```python
from build123d import *

# Parameters (mm, degrees)
SKETCH1_W           = 24.999989911
SKETCH1_H           = 10.457138345
SKETCH1_W_2         = 49.999979697
SKETCH1_H_2         = 10.999995004
BOSS_EXTRUDE1_DEPTH = 6


with BuildPart() as part:
    # Sketch1 → Boss-Extrude1 (new body)
    with BuildSketch(Plane.XY):
        Polygon((-65.562023318, 106.501824812), (-13.869587203, 106.501824812), (-8.869589203, 111.501822737), (-8.86958929, 177.416081581), (-13.869587182, 182.416079474), (-65.562023318, 182.416079474), (-70.562021318, 177.416081474), (-70.562021318, 111.501822812), align=None)
        with Locations((-39.715805178, 122.080389652)):
            Rectangle(SKETCH1_W, SKETCH1_H, mode=Mode.SUBTRACT)
        with Locations((-39.715804889, 167.108942347)):
            Rectangle(SKETCH1_W_2, SKETCH1_H_2, mode=Mode.SUBTRACT)
        Polygon((-64.027895413, 142.720286351), (-63.562021318, 142.658952863), (-63.096147223, 142.720286351), (-62.662021678, 142.90010704), (-62.289229621, 143.186160446), (-62.003176215, 143.558952503), (-61.823355526, 143.993078048), (-61.762022038, 144.458952143), (-61.823355526, 144.924826238), (-62.003176215, 145.358951783), (-62.289229621, 145.73174384), (-62.662021678, 146.017797246), (-63.096147223, 146.197617935), (-63.562021318, 146.258951423), (-64.027895413, 146.197617935), (-64.462020958, 146.017797246), (-64.834813015, 145.73174384), (-65.120866421, 145.358951783), (-65.30068711, 144.924826238), (-65.362020598, 144.458952143), (-65.30068711, 143.993078048), (-65.120866421, 143.558952503), (-64.834813015, 143.186160446), (-64.462020958, 142.90010704), align=None, mode=Mode.SUBTRACT)
        Polygon((-15.869589241, 146.258951423), (-16.335463335, 146.197617935), (-16.769588881, 146.017797246), (-17.142380938, 145.73174384), (-17.428434344, 145.358951783), (-17.608255032, 144.924826238), (-17.669588521, 144.458952143), (-17.608255032, 143.993078048), (-17.428434344, 143.558952503), (-17.142380938, 143.186160446), (-16.769588881, 142.90010704), (-16.335463335, 142.720286351), (-15.869589241, 142.658952863), (-15.403715146, 142.720286351), (-14.969589601, 142.90010704), (-14.596797544, 143.186160446), (-14.310744137, 143.558952503), (-14.130923449, 143.993078048), (-14.069589961, 144.458952143), (-14.130923449, 144.924826238), (-14.310744137, 145.358951783), (-14.596797544, 145.73174384), (-14.969589601, 146.017797246), (-15.403715146, 146.197617935), align=None, mode=Mode.SUBTRACT)
        Polygon((-37.977139407, 111.967698907), (-38.156960096, 112.401824452), (-38.443013502, 112.774616509), (-38.815805559, 113.060669915), (-39.249931104, 113.240490604), (-39.715805199, 113.301824092), (-40.181679294, 113.240490604), (-40.615804839, 113.060669915), (-40.988596896, 112.774616509), (-41.274650303, 112.401824452), (-41.454470991, 111.967698907), (-41.515804479, 111.501824812), (-41.454470991, 111.035950717), (-41.274650303, 110.601825172), (-40.988596896, 110.229033115), (-40.615804839, 109.942979709), (-40.181679294, 109.76315902), (-39.715805199, 109.701825532), (-39.249931104, 109.76315902), (-38.815805559, 109.942979709), (-38.443013502, 110.229033115), (-38.156960096, 110.601825172), (-37.977139407, 111.035950717), (-37.915805919, 111.501824812), align=None, mode=Mode.SUBTRACT)
        Polygon((-37.977139407, 176.950205359), (-37.915805919, 177.416079454), (-37.977139407, 177.881953549), (-38.156960096, 178.316079094), (-38.443013502, 178.688871151), (-38.815805559, 178.974924557), (-39.249931104, 179.154745246), (-39.715805199, 179.216078734), (-40.181679294, 179.154745246), (-40.615804839, 178.974924557), (-40.988596896, 178.688871151), (-41.274650303, 178.316079094), (-41.454470991, 177.881953549), (-41.515804479, 177.416079454), (-41.454470991, 176.950205359), (-41.274650303, 176.516079814), (-40.988596896, 176.143287757), (-40.615804839, 175.857234351), (-40.181679294, 175.677413662), (-39.715805199, 175.616080174), (-39.249931104, 175.677413662), (-38.815805559, 175.857234351), (-38.443013502, 176.143287757), (-38.156960096, 176.516079814), align=None, mode=Mode.SUBTRACT)
        Polygon((-55.181679294, 134.720286351), (-54.715805199, 134.658952863), (-54.249931104, 134.720286351), (-53.815805559, 134.90010704), (-53.443013502, 135.186160446), (-53.156960096, 135.558952503), (-52.977139407, 135.993078048), (-52.915805919, 136.458952143), (-52.977139407, 136.924826238), (-53.156960096, 137.358951783), (-53.443013502, 137.73174384), (-53.815805559, 138.017797246), (-54.249931104, 138.197617935), (-54.715805199, 138.258951423), (-55.181679294, 138.197617935), (-55.615804839, 138.017797246), (-55.988596896, 137.73174384), (-56.274650303, 137.358951783), (-56.454470991, 136.924826238), (-56.515804479, 136.458952143), (-56.454470991, 135.993078048), (-56.274650303, 135.558952503), (-55.988596896, 135.186160446), (-55.615804839, 134.90010704), align=None, mode=Mode.SUBTRACT)
        Polygon((-23.156960096, 137.358951783), (-23.443013502, 137.73174384), (-23.815805559, 138.017797246), (-24.249931104, 138.197617935), (-24.715805199, 138.258951423), (-25.181679294, 138.197617935), (-25.615804839, 138.017797246), (-25.988596896, 137.73174384), (-26.274650303, 137.358951783), (-26.454470991, 136.924826238), (-26.515804479, 136.458952143), (-26.454470991, 135.993078048), (-26.274650303, 135.558952503), (-25.988596896, 135.186160446), (-25.615804839, 134.90010704), (-25.181679294, 134.720286351), (-24.715805199, 134.658952863), (-24.249931104, 134.720286351), (-23.815805559, 134.90010704), (-23.443013502, 135.186160446), (-23.156960096, 135.558952503), (-22.977139407, 135.993078048), (-22.915805919, 136.458952143), (-22.977139407, 136.924826238), align=None, mode=Mode.SUBTRACT)
    extrude(amount=BOSS_EXTRUDE1_DEPTH)


solid = part.part
```
Can you work these out from the model? Positions are in its coordinate system, mm. A direction names the side the tool comes from. Coordinates: 2 decimals unless noted, no trailing zeros. Loops run counter-clockwise (first coordinate to the right, second up) from the corner with the lowest first, then second, coordinate; pieces in that order, holes last. Notation, with made-up numbers: (32, 5.5) -> (88, 5.5) arc R27 ccw to (88, 28.5) -> close; hole circle Ø8 at (-9, 48.5). An arc over 180 degrees is marked (long way). Put each result on its own line as item: value. Start each with the question number.
Q1. Thinking about a two-plate mould opening in Y: for faces 1 (the face through (-68.03, 179.95, 2.96)), 2 (the face through (-40, 172.609, 3)), 3 (the face through (-40, 145, 0)), 4 (the face through (-27.216, 122, 3)), which applies, pulls with the +Y half, pulls with the -Y half, needs draft (parallel to the pull), parting line crosses it, or undercut?
Q2. I want a section at C-C (y = 170). Write out the boundary of the cut face in (x, z).
Q3. I want a section at D-D (z = 2.25). Count the separate pieces of the cut face and the enclosed holes in it, plus the area to 3 significant figures.
Q4. I want a section at B-B (x = -51). Write out the boundary of the cut face in (y, z).
Q5. For faces 5 (the face through (-52.216, 122, 3)), 6 (the face through (-40, 145, 6)), which set-ups out of +Z, -Z, +X, -X, +Y, -Y let a thin tool reach every point of the face, with its end or its side?
Q6. I want a section at A-A (x = -19.5). Write out the boundary of the cut face in (y, z), plus the area to 3 significant figures.
Q7. If I drill on line 1 (Y direction, x = -26, z = 4.75); line 2 (Y direction, x = -36.5, z = 3.55); line 3 (X direction, y = 166, z = 0.4), over which ranges is the centre line in solid material (lowest first)? Write a range as [from, to].
Q8. I'm going to push a flat-ended pin straight in: P1, Ø5, axis at x = -47.5, y = 164.5, coming from the -Z side. Where does the tip first touch, or does it pass through?
Taken from the geometry:
1. face 1: pulls with the +Y half
1. face 2: undercut
1. face 3: needs draft
1. face 4: undercut
2. outline: (-70.56, 0) -> (-64.72, 0) -> (-64.72, 6) -> (-70.56, 6) -> close; (-14.72, 0) -> (-8.87, 0) -> (-8.87, 6) -> (-14.72, 6) -> close
3. separate pieces: 1
3. enclosed holes: 8
3. area: 3,760 mm2
4. outline: (106.5, 0) -> (116.85, 0) -> (116.85, 6) -> (106.5, 6) -> close; (127.31, 0) -> (161.61, 0) -> (161.61, 6) -> (127.31, 6) -> close; (172.61, 0) -> (182.42, 0) -> (182.42, 6) -> (172.61, 6) -> close
5. face 5: +Z, -Z
5. face 6: +Z, +X, -X, +Y, -Y
6. outline: (106.5, 0) -> (161.61, 0) -> (161.61, 6) -> (106.5, 6) -> close; (172.61, 0) -> (182.42, 0) -> (182.42, 6) -> (172.61, 6) -> close
6. area: 389 mm2
7. line 1: y = [106.5, 135.2], [137.72, 161.61], [172.61, 182.42]
7. line 2: y = [106.5, 116.85], [127.31, 161.61], [172.61, 182.42]
7. line 3: x = [-70.56, -64.72], [-14.72, -8.87]
8. P1: passes through
